The listing builds one solid part. Answer for the finished solid, in the listing's coordinates (mm). A direction names the side the tool comes from. Coordinates: 2 decimals unless noted, no trailing zeros. Loops run counter-clockwise (first coordinate to the right, second up) from the corner with the lowest first, then second, coordinate; pieces in that order, holes last. Notation, with made-up numbers: (43, 9) - (61, 9) arc R24 ccw to (61, 33) - close; hole circle Ø8 at (75, 51). An arc over 180 degrees is marked (long way). Write each question's results on one line, items separated by ' | '. Start each with the question number.
(1) Find section C-C on y = 8. Determine the outline of the cut face in (x, z), then the cut area to 3 significant figures.
(2) Find section A-A on z = -14. Determine the outline of the cut face in (x, y) (3 decimals), then the cut area to 3 significant figures.
(3) Find section B-B on x = 43. Determine the outline of the cut face in (y, z), then the cut area to 3 significant figures.
(4) Determine the mould class of faces 4 (the flat face through (43, 13.85, 10)), 5 (the cylindrical face through (33.23, 20.45, 0.13)), 6 (the cylindrical face through (8.902, 11.351, -13.837)), 7 (the cylindrical face through (33.23, 2.95, 0.13)) for opening direction X: released by +X, released by -X, zero draft, split by the parting line, or undercut.
(5) Consider line 1 (Y direction, x = 31.8, z = -5); line 2 (Y direction, x = 33, z = -0.5); line 3 (Y direction, x = 11.2, z = -13) (3 decimals). Determine where each line is inside the solid, lowest interval first. Write a range as from..to.
(6) For faces 1 (the flat face through (44.6, 11, 10)), 2 (the flat face through (11, 9.45, -15)), 3 (the flat face through (11, 13.05, -15)), determine the directions among +Z, -Z, +X, -X, +Y, -Y from which every point of the face is accessible in a straight line to the end or side of a thin tool.
(7) Given pin 1 Ø0.9 at (x, z) = (10.5, -14.5) entering from -Y; pin 2 Ø6 at (x, z) = (8, 13) entering from +Y; pin 3 Ø5 at (x, y) = (31.8, 2.5) entering from +Z, each flat-ended and moving along its own axis, determine where each tip first touches the part or whether it passes through.
from build123d import *

# Parameters (mm, degrees)
ESBO_O1_W                = 64.2
ESBO_O1_H                = 22.5
RESSALTO_EXTRUS_O1_DEPTH = 9.4
ESBO_O2_R                = 2.3
RESSALTO_EXTRUS_O2_DEPTH = 9
CORTE_EXTRUS_O1_DEPTH    = 7.9
ESBO_O4_R                = 1.5
CORTE_EXTRUS_O2_DEPTH    = 19.8
FILETE1_R                = 2.3
ESBO_O5_W                = 2.8
ESBO_O5_H                = 5.2
RESSALTO_EXTRUS_O3_DEPTH = 1.85


with BuildPart() as part:
    # Esboço1 → Ressalto-extrusão1 (new body, symmetric)
    with BuildSketch(Plane.XY):
        with Locations((32.1, 11.25)):
            Rectangle(ESBO_O1_W, ESBO_O1_H)
    extrude(amount=RESSALTO_EXTRUS_O1_DEPTH, both=True)

    # Esboço2 → Ressalto-extrusão2 (add)
    with BuildSketch(Plane.XY.offset(9.4)):
        with Locations((11.2, 11.25)):
            Circle(ESBO_O2_R)
    ressalto_extrus_o2 = extrude(amount=RESSALTO_EXTRUS_O2_DEPTH)

    # Esboço3 → Corte-extrusão1 (cut)
    with BuildSketch(Plane.XY.offset(18.4)):
        with BuildLine():
            Line((9.768217894, 13.05), (12.631782106, 13.05))
            ThreePointArc((12.631782106, 13.05), (11.2, 13.55), (9.768217894, 13.05))
        make_face()
        with BuildLine():
            Line((12.631782106, 9.45), (9.768217894, 9.45))
            ThreePointArc((9.768217894, 9.45), (11.2, 8.95), (12.631782106, 9.45))
        make_face()
    corte_extrus_o1 = extrude(amount=-CORTE_EXTRUS_O1_DEPTH, mode=Mode.SUBTRACT)

    # Esboço4 → Corte-extrusão2 (cut, through all)
    with BuildSketch(Plane.XY.offset(9.4)):
        with Locations((31.8, 20)):
            Circle(ESBO_O4_R)
        with Locations((31.8, 2.5)):
            Circle(ESBO_O4_R)
    extrude(amount=-CORTE_EXTRUS_O2_DEPTH, mode=Mode.SUBTRACT)

    # Esboço6 → Furo roscado de M2.51 (revolve, cut)
    with BuildSketch(Plane(origin=(11.2, 11.25, 18.4), x_dir=(0, -1, 0), z_dir=(1, 0, 0))):
        Polygon((0, 0), (0, 7.865882135), (1.025, 7.25), (1.025, 0), align=None)
    furo_roscado_de_m2_51 = revolve(axis=Axis((11.2, 11.25, 24.75), (0, 0, -1)), mode=Mode.SUBTRACT)

    # Espelhar1: Ressalto-extrusão2, Corte-extrusão1, Furo roscado de M2.51 across plane
    add(ressalto_extrus_o2.mirror(Plane.XY))
    add(corte_extrus_o1.mirror(Plane.XY), mode=Mode.SUBTRACT)
    add(furo_roscado_de_m2_51.mirror(Plane.XY), mode=Mode.SUBTRACT)

    # Filete1
    filete1_edges = [part.edges().sort_by_distance(p)[0] for p in [
        (0, 22.5, 0),
        (0, 0, 0),
    ]]
    fillet(filete1_edges, radius=FILETE1_R)

    # Esboço5 → Ressalto-extrusão3 (add)
    with BuildSketch(Plane.XY.offset(9.4)):
        with Locations((43.2, 11.25)):
            Rectangle(ESBO_O5_W, ESBO_O5_H)
    extrude(amount=RESSALTO_EXTRUS_O3_DEPTH)


solid = part.part
Values:
1) outline: (0, -9.4) - (64.2, -9.4) - (64.2, 9.4) - (0, 9.4) - close | area: 1,210 mm²
2) outline: (9.768, 9.45) - (12.632, 9.45) arc R2.3 ccw to (12.632, 13.05) - (9.768, 13.05) arc R2.3 ccw to start; hole circle Ø2.05 at (11.2, 11.25) | area: 11.4 mm²
3) outline: (0, -9.4) - (22.5, -9.4) - (22.5, 9.4) - (13.85, 9.4) - (13.85, 11.25) - (8.65, 11.25) - (8.65, 9.4) - (0, 9.4) - close | area: 433 mm²
4) face 4: zero draft | face 5: undercut | face 6: split by the parting line | face 7: undercut
5) line 1: y = 0..1, 4..18.5, 21.5..22.5 | line 2: y = 0..1.6, 3.4..19.1, 20.9..22.5 | line 3: y = 9.45..10.225, 12.275..13.05
6) face 1: +Z, +X, +Y, -Y | face 2: -Z, +X, -X, -Y | face 3: -Z, +X, -X, +Y
7) pin 1: stops at y = 9.45 | pin 2: stops at y = 13.05 | pin 3: stops at z = 9.4
